Could you check a few things on this drawing? It's one solid part, dimensions in mm from its lowest x, y, z. Round coordinates to 2 decimals unless told otherwise and drop trailing zeros. Loops run counter-clockwise (first coordinate to the right, second up) from the corner with the lowest first, then second, coordinate; pieces in that order, holes last. Notation, with made-up numbers: M 30,5 L 35,5 A21 ccw 35,26 Z; hole C 9.25,3.5 d10. An arc over 180 degrees is marked long. Answer as a JSON object with one key per item and string values.
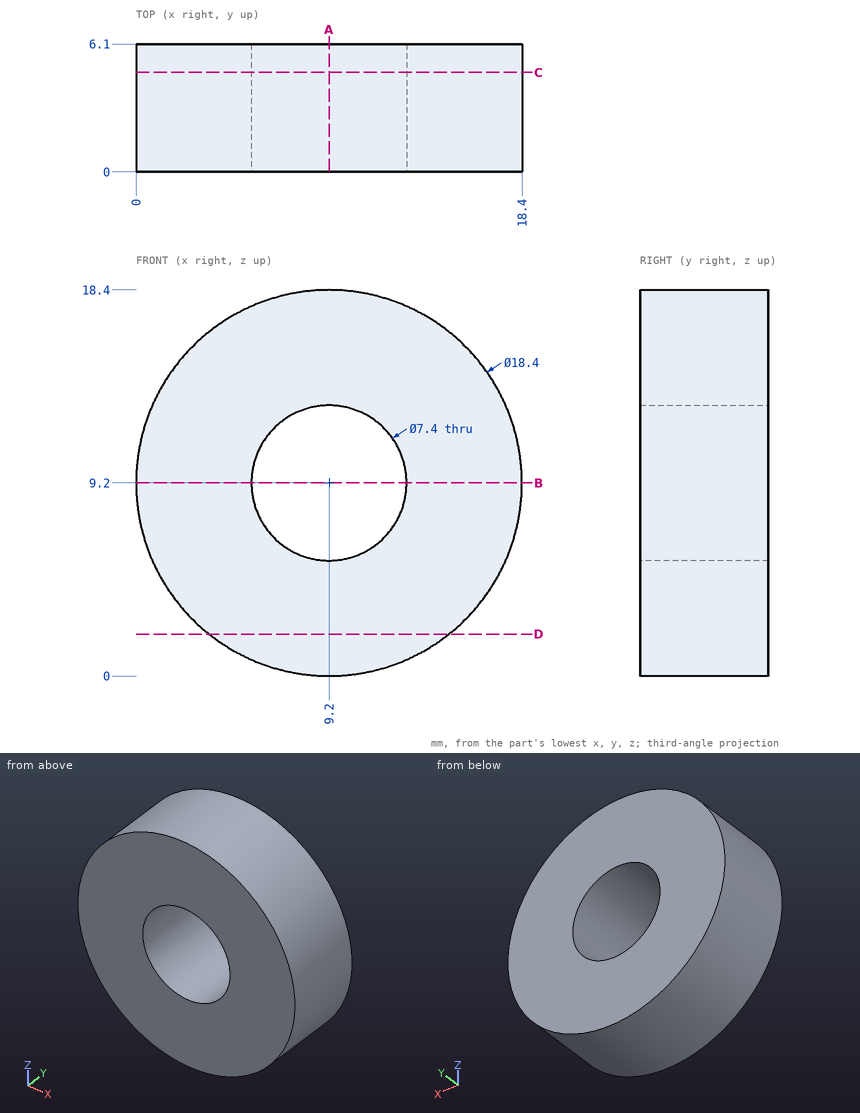
Item 1: I want a section at C-C, the plane y = 4.75. Please give me the cut outline in (x, z), then the cut area to 3 significant figures.
Resolved:
{"outline": "C 9.2,9.2 d18.4; hole C 9.2,9.2 d7.4", "area": "223 mm²"}
Item 2: I want a section at A-A, the plane x = 9.2. Please give me the cut outline in (y, z), then the cut area to 3 significant figures.
Resolved:
{"outline": "M 0,0 L 6.1,0 L 6.1,5.5 L 0,5.5 Z; M 0,12.9 L 6.1,12.9 L 6.1,18.4 L 0,18.4 Z", "area": "67.1 mm²"}
Item 3: I want a section at D-D, the plane z = 2. Please give me the cut outline in (x, y), then the cut area to 3 significant figures.
Resolved:
{"outline": "M 3.47,0 L 14.93,0 L 14.93,6.1 L 3.47,6.1 Z", "area": "69.9 mm²"}
Item 4: Please list where these lines run through material, in increasing order: probe 1 along Z at (x, y) = (9.2, 3); probe 2 along X at (y, z) = (4.75, 10.5). Write a range as from..to.
Resolved:
{"probe 1": "0..5.5, 12.9..18.4", "probe 2": "0.09..5.74, 12.66..18.31"}
Item 5: I'm going to push flat-ended pins straight in: pin 1 Ø6.5 at (x, z) = (9.2, 9.2) entering from +Y (3 decimals); pin 2 Ø2 at (y, z) = (1, 7.5) entering from +X; pin 3 Ø3 at (y, z) = (2.5, 3.5) entering from -X; pin 4 Ø2 at (x, y) = (12, 2.5) entering from -Z. Where does each tip first touch, or does it pass through?
Resolved:
{"pin 1": "through", "pin 2": "x = 18.37", "pin 3": "x = 1.01", "pin 4": "z = 0.18"}
Item 6: I want a section at B-B, the plane z = 9.2. Please give me the cut outline in (x, y), then the cut area to 3 significant figures.
Resolved:
{"outline": "M 0,0 L 5.5,0 L 5.5,6.1 L 0,6.1 Z; M 12.9,0 L 18.4,0 L 18.4,6.1 L 12.9,6.1 Z", "area": "67.1 mm²"}
